from build123d import *

# Parameters (mm, degrees)
SKIZZE1_W                       = 110
SKIZZE1_H                       = 100
AUFSATZ_LINEAR_AUSTRAGEN1_DEPTH = 15
SKIZZE2_R                       = 33.5
SCHNITT_LINEAR_AUSTRAGEN1_DEPTH = 7.5
SKIZZE3_R                       = 26
SCHNITT_LINEAR_AUSTRAGEN2_DEPTH = 7.5
SKIZZE4_R                       = 2.1
SCHNITT_LINEAR_AUSTRAGEN3_DEPTH = 10
SKIZZE5_R                       = 1.25
SCHNITT_LINEAR_AUSTRAGEN5_DEPTH = 10
VERRUNDUNG1_R                   = 50


with BuildPart() as part:
    # Skizze1 → Aufsatz-Linear austragen1 (new body)
    with BuildSketch(Plane.XY):
        with Locations((55, 50)):
            Rectangle(SKIZZE1_W, SKIZZE1_H)
    extrude(amount=AUFSATZ_LINEAR_AUSTRAGEN1_DEPTH)

    # Skizze2 → Schnitt-Linear austragen1 (cut)
    with BuildSketch(Plane.XY.offset(15)):
        with Locations((55, 50)):
            Circle(SKIZZE2_R)
    extrude(amount=-SCHNITT_LINEAR_AUSTRAGEN1_DEPTH, mode=Mode.SUBTRACT)

    # Skizze3 → Schnitt-Linear austragen2 (cut)
    with BuildSketch(Plane(origin=(0, 0, 0), x_dir=(-1, 0, 0), z_dir=(0, 0, -1))):
        with Locations((-55, 50)):
            Circle(SKIZZE3_R)
    extrude(amount=-SCHNITT_LINEAR_AUSTRAGEN2_DEPTH, mode=Mode.SUBTRACT)

    # Skizze4 → Schnitt-Linear austragen3 (cut)
    with BuildSketch(Plane.XZ):
        with Locations(Location((25, 7.5, 0), (0, 0, 270))):
            Circle(SKIZZE4_R)
        with Locations(Location((85, 7.5, 0), (0, 0, 270))):
            Circle(SKIZZE4_R)
        with Locations(Location((55, 7.5, 0), (0, 0, 270))):
            Circle(SKIZZE4_R)
    extrude(amount=-SCHNITT_LINEAR_AUSTRAGEN3_DEPTH, mode=Mode.SUBTRACT)

    # Skizze5 → Schnitt-Linear austragen5 (cut)
    with BuildSketch(Plane.XY.offset(15)):
        with Locations((55, 96)):
            Circle(SKIZZE5_R)
        with Locations((90.964248194, 78.680530886)):
            Circle(SKIZZE5_R)
        with Locations((99.84668396, 39.764037038)):
            Circle(SKIZZE5_R)
        with Locations((74.958651999, 8.555432076)):
            Circle(SKIZZE5_R)
        with Locations((35.041348001, 8.555432076)):
            Circle(SKIZZE5_R)
        with Locations((10.15331604, 39.764037038)):
            Circle(SKIZZE5_R)
        with Locations((19.035751806, 78.680530886)):
            Circle(SKIZZE5_R)
    extrude(amount=-SCHNITT_LINEAR_AUSTRAGEN5_DEPTH, mode=Mode.SUBTRACT)

    # Verrundung1
    verrundung1_edges = [part.edges().sort_by_distance(p)[0] for p in [
        (0, 100, 7.5),
        (110, 100, 7.5),
    ]]
    fillet(verrundung1_edges, radius=VERRUNDUNG1_R)


solid = part.part
Can you work these out from the model? Positions are in its coordinate system, mm. A direction names the side the tool comes from. Round coordinates to 2 decimals unless told otherwise and drop trailing zeros. Loops run counter-clockwise (first coordinate to the right, second up) from the corner with the lowest first, then second, coordinate; pieces in that order, holes last. Notation, with made-up numbers: (22, 72) - (41, 72) arc R5 ccw to (41, 79) - close; hole circle Ø4 at (11, -23). An arc over 180 degrees is marked (long way). Answer in a Markdown table with one row per item. Add a question column.
Q1. I want a section at C-C on z = 3. List the corners of the cut face in (x, y) for me.
Q2. We'd pull the mould along Y, two halves only. Please class faces 4 (the cylindrical face through (94.964, 85.742, 7.605)), 5 (the flat face through (91, 79, 5)), 6 (the flat face through (30, 40, 0)), 7 (the cylindrical face through (73.71, 8.61, 10.07)): pulls with the +Y half, pulls with the -Y half, needs draft (parallel to the pull), parting line crosses it, or undercut.
Q3. I need wall thicknesses on L1, parallel to X at y = 2.25, z = 7.5; L2, parallel to X at y = 39, z = 10.75; L3, parallel to Y at x = 55.5, z = 4.75. Which ranges of each line are inside material? Lowest first, please.
Q4. I want a section at D-D on y = 58.5. List the corners of the cut face in (x, z) for me, and give its area (3 significant figures).
Q5. I want a section at B-B on y = 34. List the corners of the cut face in (x, z) for me.
Q6. For pin 1 Ø1.2 at (x, y) = (9.5, 40.5) entering from +Z; pin 2 Ø3.5 at (x, z) = (85, 7.5) entering from +Y; pin 3 Ø1.5 at (x, z) = (84.5, 7) entering from +Y; pin 4 Ø12 at (x, y) = (50.5, 25) entering from +Z, each with a flat end and sliding along its axis, tell me the tip position at first contact or that it passes through.
Q7. Which directions (+Z, -Z, +X, -X, +Y, -Y) give clear straight access to the entire face, cutting with the end or side of a thin tool? Please do faces 1 (the cylindrical face through (52.95, 4.93, 7.96)), 2 (the flat face through (66, 17, 15)), 3 (the flat face through (10, 40, 5)).
Q8. I want a section at A-A on x = 55. List the corners of the cut face in (y, z) for me, and give its area (4 significant figures).
A:
| question | item | result |
|---|---|---|
| 1 | outline | (0, 0) - (110, 0) - (110, 50) arc R50 ccw to (60, 100) - (50, 100) arc R50 ccw to (0, 50) - close; hole circle Ø52 at (55, 50) |
| 2 | face 4 | pulls with the +Y half |
| 2 | face 5 | undercut |
| 2 | face 6 | needs draft |
| 2 | face 7 | undercut |
| 3 | L1 | 0 to 22.9, 27.1 to 52.9, 57.1 to 82.9, 87.1 to 110 |
| 3 | L2 | 0 to 9.16, 11.14 to 23.36, 86.64 to 98.86, 100.84 to 110 |
| 3 | L3 | 0 to 24, 76 to 100 |
| 4 | outline | (0.73, 0) - (30.43, 0) - (30.43, 7.5) - (22.6, 7.5) - (22.6, 15) - (0.73, 15) - close; (79.57, 0) - (109.27, 0) - (109.27, 15) - (87.4, 15) - (87.4, 7.5) - (79.57, 7.5) - close |
| 4 | area | 774 mm^2 |
| 5 | outline | (0, 0) - (34.51, 0) - (34.51, 7.5) - (25.57, 7.5) - (25.57, 15) - (0, 15) - close; (75.49, 0) - (110, 0) - (110, 15) - (84.43, 15) - (84.43, 7.5) - (75.49, 7.5) - close |
| 6 | pin 1 | z = 15 |
| 6 | pin 2 | y = 94.27 |
| 6 | pin 3 | y = 94 |
| 6 | pin 4 | z = 7.5 |
| 7 | face 1 | -Y |
| 7 | face 2 | +Z, +X, -X, +Y, -Y |
| 7 | face 3 | +Z |
| 8 | outline | (0, 0) - (24, 0) - (24, 7.5) - (16.5, 7.5) - (16.5, 15) - (0, 15) - (0, 9.6) - (10, 9.6) - (10, 5.4) - (0, 5.4) - close; (76, 0) - (100, 0) - (100, 15) - (97.25, 15) - (97.25, 5) - (94.75, 5) - (94.75, 15) - (83.5, 15) - (83.5, 7.5) - (76, 7.5) - close |
| 8 | area | 540.5 mm^2 |
